The model under review builds one solid part; all positions refer to its coordinate system, in mm. A direction names the side the tool comes from. Round coordinates to 2 decimals unless told otherwise and drop trailing zeros. Write each loop counter-clockwise with the first axis right and the second up, starting at its lowest first coordinate (ties: lowest second). Pieces come first, ordered by that corner, then holes. Notation, with made-up numbers: M -7,86 L 49,86 A20 ccw 49,102 Z; hole C -3.5,17 d5. An arc over 180 degrees is marked long. One line per item, written item: value. Start each with the question number.
1) Wall thickness on probe 1 along Z at (x, y) = (0, 11.25); probe 2 along X at (y, z) = (15.75, 1); probe 3 along X at (y, z) = (9.75, -1): over which ranges is each line inside the solid? List them lowest first.
2) For P1, Ø1, axis at x = 13.5, z = 10.5, coming from the +Y side; P2, Ø3, axis at x = -3.43, z = 10.56, coming from the +Y side; P3, Ø1.5, axis at x = 1, y = 7, coming from the -Z side, all flat-tipped, find the tip position at first contact; note any pin that passes through.
3) Mouldability with a two-part tool opening along Z and no side actions: class faces 1 (the face through (-4.678, 13.589, -7.338)), 2 (the face through (-4, 0, -4)), 3 (the face through (-3.14, 4.61, -9.24)) as +Z half, -Z half, draft (parallel to the pull), parting line (faces both ways), or undercut.
4) Tool access review of faces 4 (the face through (3.88, 1.97, 2.28)), 5 (the face through (-2.2, 19, -2.2)): name each direction out of +Z, -Z, +X, -X, +Y, -Y from which nothing blocks a thin tool from reaching the whole face with its end or side.
5) Take a section at B-B, the plane y = 13.75. Write out the cut boundary in (x, z), and give its area (3 significant figures).
Autodesk Inventor part; units mm, degrees
ref_plane "YZ Plane" through (0, 0, 0) normal (1, 0, 0) x (0, 1, 0)
ref_plane "XZ Plane" through (0, 0, 0) normal (0, 1, 0) x (-1, 0, 0)
ref_plane "XY Plane" through (0, 0, 0) normal (0, 0, 1) x (1, 0, 0)
sketch "Sketch1" plane through (0, 0, 0) normal (0, 1, 0) x (-1, 0, 0)
  circle A0 centre (0, 0) radius 18
  line L0 (10.3065, -1.0922) -> (4.2236, -9.4646)
  line L1 (2.1462, -10.1396) -> (-7.6962, -6.9416)
  line L2 (-8.9801, -5.1744) -> (-8.9801, 5.1744)
  line L3 (-7.6962, 6.9416) -> (2.1462, 10.1396)
  line L4 (4.2236, 9.4646) -> (10.3065, 1.0922)
  circle A1 centre (3.4301, 10.5567) radius 1.35
  circle A2 centre (11.1, 0) radius 1.35
  circle A3 centre (-8.9801, 6.5244) radius 1.35
  circle A4 centre (-8.9801, -6.5244) radius 1.35
  circle A5 centre (3.4301, -10.5567) radius 1.35
  arc A6 (11.0179, 1.3475) -> (4.6863, 10.0622) centre (0, 0) ccw
  arc A7 (4.6863, -10.0622) -> (11.0179, -1.3475) centre (0, 0) ccw
  arc A8 (-8.1216, -7.5663) -> (2.1232, -10.8951) centre (0, 0) ccw
  arc A9 (2.1232, 10.8951) -> (-8.1216, 7.5663) centre (0, 0) ccw
  arc A10 (-9.7057, 5.386) -> (-9.7057, -5.386) centre (0, 0) ccw
  dimension "d0" = 36
  dimension "d2" = 2.7
  dimension "d3" = 2.7
  dimension "d4" = 2.7
  dimension "d5" = 2.7
  dimension "d6" = 2.7
extrude "Extrusion1" add sketch "Sketch1" along normal blind 19 contours A0 | A2 A7 A5 L0 | L0 A5 L1 A4 L2 A3 L3 A1 L4 A2 | A2 | A5 | L4 A1 A6 A2 | A5 A8 A4 L1 | A1 | A4 | L3 A3 A9 A1 | A3 | A10 A3 L2 A4
sketch "Sketch3" plane through (0, 0, 0) normal (0, -1, 0) x (1, 0, 0)
  circle A0 centre (0, 0) radius 18
  line L0 (-5.1962, 0) -> (-2.5981, 4.5)
  line L1 (-2.5981, 4.5) -> (2.5981, 4.5)
  line L2 (2.5981, 4.5) -> (5.1962, 0)
  line L3 (5.1962, 0) -> (2.5981, -4.5)
  line L4 (2.5981, -4.5) -> (-2.5981, -4.5)
  line L5 (-2.5981, -4.5) -> (-5.1962, 0)
  dimension "d23" = 9
extrude "Extrusion3" cut sketch "Sketch3" against normal blind 4 contours L0 L1 L2 L3 L4 L5
sketch "Sketch4" plane through (0, 4, 0) normal (0, -1, 0) x (1, 0, 0)
  circle A0 centre (0, 0) radius 2.75
  dimension "d26" = 5.5
extrude "Extrusion4" cut sketch "Sketch4" against normal blind 17
chamfer "Chamfer2" distance 13 distance2 19 1 edges at (18, 19, 0) measured on face at (-12.7157, 19, -1.6553)
extrude "Extrusion5" cut sketch "Sketch1" along normal blind 14 contours A2 | A5 | A1 | A4 | A3
equation "\"BendRadius\" = Thickness"
equation "\"BendReliefWidth\" = Thickness"
equation "\"BendReliefDepth\" = 0.5 * Thickness"
equation "\"CornerReliefSize\" = 4 * Thickness"
equation "\"MinimumRemnant\" = 2 * Thickness"
equation "\"TransitionRadius\" = BendRadius"
equation "\"JacobiRadiusSize\" = BendRadius"
equation "\"GapSize\" = Thickness"
properties part number "motorSupportShaft"
Checked values:
1. probe 1: z = -10.3 to -2.75, 2.75 to 10.3
1. probe 2: x = -7.15 to -2.56, 2.56 to 7.15
1. probe 3: x = -10.19 to -2.56, 2.56 to 11.29
2. P1: stops at y = 2.04
2. P2: stops at y = 12.27
2. P3: stops at z = -13.69
3. face 1: parting line
3. face 2: draft
3. face 3: undercut
4. face 4: -Y
4. face 5: +Z, -Z, +X, -X, +Y
5. outline: C 0,0 d17.19; hole C 0,0 d5.5
5. area: 208 mm2
